from build123d import *

# Parameters (mm, degrees)
F0_W     = 60
F0_H     = 168
F1_DEPTH = 100
F2_T     = -1.5
F3_W     = 57
F3_H     = 1.5
F4_DEPTH = 98.5
F5_R     = 2
F6_R     = 2.5


with BuildPart() as f1:
    # F0 (on Top) → F1 (new body)
    with BuildSketch(Plane.XY):
        Rectangle(F0_W, F0_H)
    extrude(amount=F1_DEPTH)

    # F2
    f2_openings = [f1.faces().sort_by_distance(p)[0] for p in [
        (0, 0, 100),
    ]]
    offset(amount=F2_T, openings=f2_openings)

    # F3 (on face) → F4 (join, through all)
    with BuildSketch(Plane.XY.offset(1.5)):
        with Locations((0, 14.9535381934)):
            Rectangle(F3_W, F3_H)
        with Locations((0, -35.4550533295)):
            Rectangle(F3_W, F3_H)
    extrude(amount=F4_DEPTH)

    # F5
    f5_edges = [f1.edges().sort_by_distance(p)[0] for p in [
        (-28.5, -82.5, 50.75),
        (-28.5, 14.203538, 50.75),
        (-28.5, 82.5, 50.75),
        (28.5, 82.5, 50.75),
        (28.5, 15.703538, 50.75),
        (28.5, -82.5, 50.75),
        (28.5, 14.203538, 50.75),
        (-28.5, 15.703538, 50.75),
        (-28.5, -36.205053, 50.75),
        (-28.5, -34.705053, 50.75),
        (28.5, -34.705053, 50.75),
        (28.5, -36.205053, 50.75),
    ]]
    fillet(f5_edges, radius=F5_R)

    # F6
    f6_edges = [f1.edges().sort_by_distance(p)[0] for p in [
        (30, -84, 50),
        (-30, -84, 50),
        (30, 84, 50),
        (-30, 84, 50),
    ]]
    fillet(f6_edges, radius=F6_R)


solid = f1.part
Work out the finished part from the listing and answer in its coordinate system (mm). A direction names the side the tool comes from. Round coordinates to 2 decimals unless told otherwise and drop trailing zeros. Order: outer loops, then holes, each group sorted by start corner. A loop starts at its lowest first (then second) coordinate and runs counter-clockwise, first axis right, second up. Notation, with made-up numbers: M 69.5,-18.75 L 91.5,-18.75 A10 cw 91.5,-3.75 Z; hole C 43,47.5 d3. An arc over 180 degrees is marked long. One line per item, written item: value.
Q1. For faces 1 (the face through (0, -84, 49)), 2 (the face through (28.5, 49, 50)), determine the directions among +Z, -Z, +X, -X, +Y, -Y from which every point of the face is accessible in a straight line to the end or side of a thin tool.
Derived:
face 1: +Z, -Z, +X, -X, -Y
face 2: +Z
Q2. Find section B-B on y = 9.5. Write down the section's boundary in (x, z), then the cut area to 4 significant figures.
Derived:
outline: M -30,0 L 30,0 L 30,100 L 28.5,100 L 28.5,1.5 L -28.5,1.5 L -28.5,100 L -30,100 Z
area: 385.5 mm²
Q3. Straight lines are drawn through the part: line 1 (Y direction, x = -5, z = 11.5); line 2 (X direction, y = 12, z = 20.5); line 3 (Z direction, x = 23.5, y = -8). For each, find the intervals that lie inside material, in ascending order.
Derived:
line 1: -84 to -82.5, -36.21 to -34.71, 14.2 to 15.7, 82.5 to 84
line 2: -30 to -28.5, 28.5 to 30
line 3: 0 to 1.5
Q4. Find section A-A on z = 85.5. Give the number of separate pieces and of enclosed holes in the cut face, then the cut area to 3 significant figures.
Derived:
separate pieces: 1
enclosed holes: 3
area: 851 mm²
Q5. Find section C-C on x = 23. Write down the section's boundary in (y, z), then the cut area to 3 significant figures.
Derived:
outline: M -84,0 L 84,0 L 84,100 L 82.5,100 L 82.5,1.5 L 15.7,1.5 L 15.7,100 L 14.2,100 L 14.2,1.5 L -34.71,1.5 L -34.71,100 L -36.21,100 L -36.21,1.5 L -82.5,1.5 L -82.5,100 L -84,100 Z
area: 843 mm²
Q6. A flat-ended cylindrical pin translates along its axis: pin 1 (14.5 mm diameter, centred on x = 7, y = -10.5, fed in from +Z). Find the tip coordinate at first contact, or state that the pin passes through.
Derived:
pin 1: z = 1.5
Q7. Determine the mould class of faces 3 (the face through (-28.5, -11, 50)), 4 (the face through (30, -1, 49)), 5 (the face through (0, 82.5, 50)), 6 (the face through (-30, -1, 49)) for opening direction X: released by +X, released by -X, zero draft, split by the parting line, or undercut.
Derived:
face 3: undercut
face 4: released by +X
face 5: undercut
face 6: released by -X
